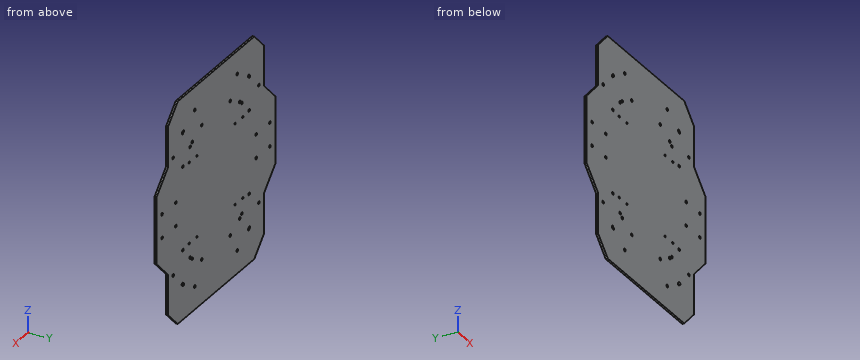
from build123d import *

# Parameters (mm, degrees)
BOSS_EXTRUDE1_DEPTH            = 3
SKETCH2_R                      = 2.05
CUT_EXTRUDE1_DEPTH             = 3
SKETCH5_R                      = 1.55
CUT_EXTRUDE2_DEPTH             = 3
LPATTERN1_COUNT                = 2
LPATTERN1_PITCH                = 120
LPATTERN1_COUNT_DIR2           = 2
LPATTERN1_PITCH_DIR2           = 120
SKETCH6_R                      = 2.05
CUT_EXTRUDE3_DEPTH             = 3
F_4_1_4_1_DIAMETER_SLOT1_DEPTH = 3


# Read off the part's stored shape, not the designer's step: Ø4.1 (4.1) Diameter Slot1
with BuildPart() as part:
    # Sketch1 → Boss-Extrude1 (new body)
    with BuildSketch(Plane(origin=(0, 0, 0), x_dir=(1, 0, 0), z_dir=(0, 1, 0))):
        Polygon((-100, 165), (-125, 140), (-125, 80), (-155, 50), (-155, -50), (-125, -80), (-125, -140), (-100, -165), (100, -165), (125, -140), (125, -80), (155, -50), (155, 50), (125, 80), (125, 140), (100, 165), align=None)
    extrude(amount=BOSS_EXTRUDE1_DEPTH)

    # Sketch2 → Cut-Extrude1 (cut)
    with BuildSketch(Plane(origin=(0, 3, 0), x_dir=(1, 0, 0), z_dir=(0, 1, 0))):
        with Locations(Location((55.344555434, 130.859581934, 0), (0, 0, 270))):
            Circle(SKETCH2_R)
        with Locations(Location((37.344555434, 99.682667397, 0), (0, 0, 270))):
            Circle(SKETCH2_R)
        with Locations(Location((37.344555434, -99.682667397, 0), (0, 0, 270))):
            Circle(SKETCH2_R)
        with Locations(Location((55.344555434, -130.859581934, 0), (0, 0, 270))):
            Circle(SKETCH2_R)
        with Locations(Location((105, 17.5, 0), (0, 0, 270))):
            Circle(SKETCH2_R)
        with Locations(Location((141, 17.5, 0), (0, 0, 270))):
            Circle(SKETCH2_R)
        with Locations(Location((105, -17.5, 0), (0, 0, 270))):
            Circle(SKETCH2_R)
        with Locations(Location((141, -17.5, 0), (0, 0, 270))):
            Circle(SKETCH2_R)
        with Locations(Location((85.655444566, -113.359581934, 0), (0, 0, 270))):
            Circle(SKETCH2_R)
        with Locations(Location((67.655444566, -82.182667397, 0), (0, 0, 270))):
            Circle(SKETCH2_R)
        with Locations(Location((85.655444566, 113.359581934, 0), (0, 0, 270))):
            Circle(SKETCH2_R)
        with Locations(Location((67.655444566, 82.182667397, 0), (0, 0, 270))):
            Circle(SKETCH2_R)
    cut_extrude1 = extrude(amount=-CUT_EXTRUDE1_DEPTH, mode=Mode.SUBTRACT)

    # Mirror1: Cut-Extrude1 across plane
    add(cut_extrude1.mirror(Plane(origin=(0, 0, 0), x_dir=(0, 0, 1), z_dir=(1, 0, 0))), mode=Mode.SUBTRACT)

    # Sketch5 → Cut-Extrude2 (cut)
    with BuildSketch(Plane(origin=(0, 3, 0), x_dir=(1, 0, 0), z_dir=(0, 1, 0))):
        with Locations(Location((50, 60, 0), (0, 0, 270))):
            Circle(SKETCH5_R)
        with Locations(Location((70, 60, 0), (0, 0, 270))):
            Circle(SKETCH5_R)
    cut_extrude2 = extrude(amount=-CUT_EXTRUDE2_DEPTH, mode=Mode.SUBTRACT)

    # LPattern1: Cut-Extrude2 2 × 2
    with Locations(*[(-j * LPATTERN1_PITCH_DIR2, 0, i * LPATTERN1_PITCH) for i in range(LPATTERN1_COUNT) for j in range(LPATTERN1_COUNT_DIR2) if (i, j) != (0, 0)]):
        add(cut_extrude2, mode=Mode.SUBTRACT)

    # Sketch6 → Cut-Extrude3 (cut)
    with BuildSketch(Plane(origin=(0, 3, 0), x_dir=(1, 0, 0), z_dir=(0, 1, 0))):
        with Locations(Location((86.620580695, 61.871843354, 0), (0, 0, 270))):
            Circle(SKETCH6_R)
        with Locations(Location((112.076424818, 87.327687477, 0), (0, 0, 270))):
            Circle(SKETCH6_R)
        with Locations((87.327687477, 112.076424818)):
            Circle(SKETCH6_R)
        with Locations(Location((61.871843354, 86.620580695, 0), (0, 0, 270))):
            Circle(SKETCH6_R)
        with Locations(Location((86.620580695, -61.871843354, 0), (0, 0, 270))):
            Circle(SKETCH6_R)
        with Locations(Location((61.871843354, -86.620580695, 0), (0, 0, 270))):
            Circle(SKETCH6_R)
        with Locations((87.405904998, -111.997966218)):
            Circle(SKETCH6_R)
        with Locations(Location((112.076424818, -87.327687477, 0), (0, 0, 270))):
            Circle(SKETCH6_R)
    cut_extrude3 = extrude(amount=-CUT_EXTRUDE3_DEPTH, mode=Mode.SUBTRACT)

    # Mirror3: Cut-Extrude3 across plane
    add(cut_extrude3.mirror(Plane(origin=(0, 0, 0), x_dir=(0, 0, 1), z_dir=(1, 0, 0))), mode=Mode.SUBTRACT)

    # Ø4.1 (4.1) Diameter Slot1 outline → Ø4.1 (4.1) Diameter Slot1 (cut)
    with BuildSketch(Plane(origin=(0, 0, 0), x_dir=(1, 0, 0), z_dir=(0, 1, 0))):
        with BuildLine():
            Line((86.83706359, 115.034776395), (86.588157233, 115.22576896))
            ThreePointArc((86.588157233, 115.22576896), (83.713821956, 114.847355542), (84.092235374, 111.973020265))
            Line((84.092235374, 111.973020265), (86.392960061, 110.207612121))
            ThreePointArc((86.392960061, 110.207612121), (89.267295338, 110.586025539), (88.88888192, 113.460360816))
            Line((88.88888192, 113.460360816), (88.639975563, 113.651353381))
            ThreePointArc((88.639975563, 113.651353381), (88.529175217, 110.415422949), (85.421153281, 111.323014333))
            ThreePointArc((85.421153281, 111.323014333), (83.740072054, 114.090231054), (86.83706359, 115.034776395))
        make_face()
        with BuildLine():
            Line((88.5093065, 113.751619279), (86.967732653, 114.934510496))
            ThreePointArc((86.967732653, 114.934510496), (87.316446435, 114.561069674), (87.561978762, 114.112992419))
            ThreePointArc((87.561978762, 114.112992419), (88.058336597, 113.991797331), (88.5093065, 113.751619279))
        make_face()
    extrude(amount=F_4_1_4_1_DIAMETER_SLOT1_DEPTH, mode=Mode.SUBTRACT)


solid = part.part
Check sheet for the modelled part. Datum: model origin and axes. Units: mm. Give positions to 0.01 mm unless a question says otherwise; leave off trailing zeros. Use one line per item in the form item = value. Start each with the question number.
1. Go/stop test with flat-tipped pins: P1, Ø2.5, axis at x = -105, z = 17.5, coming from the -Y side; P2, Ø1, axis at x = 101.5, y = 0.5, coming from the +Z side; P3, Ø6.5, axis at x = 112.08, z = -87.33, coming from the +Y side. Record where each tip stops, or that it passes through.
2. Section check A-A (y = 2). Count the separate pieces of the cut face and the enclosed holes in it, and give its area (3 significant figures).
3. Thickness scan on line 1 along Z through (x, y) = (-57, 1.6); line 2 along X through (y, z) = (2.5, -84); line 3 along Z through (x, y) = (71, 1.3). Record the ranges inside material, lowest first. Write a range as from..to.
Conclusion:
q1.P1 = through
q1.P2 = 164
q1.P3 = 3
q2.separate_pieces = 1
q2.enclosed_holes = 44
q2.area = 88,500 mm²
q3.line_1 = -165..-132.07, -129.65..129.65, 132.07..165
q3.line_2 = -125..-68.6, -66.71..66.71, 68.6..125
q3.line_3 = -165..-61.18, -58.82..58.82, 61.18..165
